from build123d import *

# Parameters (mm, degrees)
F2_SIZE = 0.5
F3_SIZE = 0.5


with BuildPart() as f1:
    # F0 (on Front) → F1 (revolve)
    with BuildSketch(Plane.XZ):
        Polygon((19, 5), (19, 0), (25, 0), (25, 15), (7, 15), (7, 5), align=None)
    revolve(axis=Axis((0, 0, 18.669182), (0, 0, 1)))

    # F2
    f2_edges = [f1.edges().sort_by_distance(p)[0] for p in [
        (-25, 0, 15),
    ]]
    chamfer(f2_edges, length=F2_SIZE)

    # F3
    f3_edges = [f1.edges().sort_by_distance(p)[0] for p in [
        (-25, 0, 0),
    ]]
    chamfer(f3_edges, length=F3_SIZE)


solid = f1.part
Could you check a few things on this model? Use its own coordinates, in mm. A direction names the side the tool comes from. Round coordinates to 2 decimals unless told otherwise and drop trailing zeros. Order: outer loops, then holes, each group sorted by start corner. A loop starts at its lowest first (then second) coordinate and runs counter-clockwise, first axis right, second up.
Q1. I'm going to push flat-ended pins straight in: P1, Ø3, axis at x = -12.5, y = -8.5, coming from the -Z side; P2, Ø1.5, axis at y = -10, z = 10.5, coming from the +X side; P3, Ø5, axis at x = 16.5, y = -17.5, coming from the -Z side; P4, Ø2, axis at x = 10, z = 3, coming from the +Y side. Where does each tip first touch, or does it pass through?
Geometry says:
P1: stops at z = 5
P2: stops at x = 23.23
P3: stops at z = 0
P4: stops at y = 23.32
Q2. Imagine slicing it at C-C, the plane z = 4.25. List the corners of the cut face in (x, y) for me.
Geometry says:
outline: circle Ø50 at (0, 0); hole circle Ø38 at (0, 0)
Q3. Imagine slicing it at A-A, the plane x = 0. List the corners of the cut face in (y, z) for me.
Geometry says:
outline: (-25, 0.5) - (-24.5, 0) - (-19, 0) - (-19, 5) - (-7, 5) - (-7, 15) - (-24.5, 15) - (-25, 14.5) - close; (7, 5) - (19, 5) - (19, 0) - (24.5, 0) - (25, 0.5) - (25, 14.5) - (24.5, 15) - (7, 15) - close
Q4. Which directions (+Z, -Z, +X, -X, +Y, -Y) give clear straight access to the entire face, cutting with the end or side of a thin tool? Please do faces 1 (the face through (8.767, -16.856, 2.465)), 2 (the face through (5.1, -5.1, 15)).
Geometry says:
face 1: -Z
face 2: +Z, +X, -X, +Y, -Y
Q5. Thinking about a two-plate mould opening in Y: for faces 3 (the face through (23.846, 7.509, 7.598)), 4 (the face through (-7, -18, 0)), 5 (the face through (0, -8, 5)), which applies, released by +Y, released by -Y, zero draft, split by the parting line, or undercut?
Geometry says:
face 3: split by the parting line
face 4: zero draft
face 5: undercut
Q6. Please list where these lines run through material, in increasing order: probe 1 along Y at (x, z) = (0, 13); probe 2 along Z at (x, y) = (11.5, -4.5); probe 3 along X at (y, z) = (2, 1).
Geometry says:
probe 1: y = -25 to -7, 7 to 25
probe 2: z = 5 to 15
probe 3: x = -24.92 to -18.89, 18.89 to 24.92
